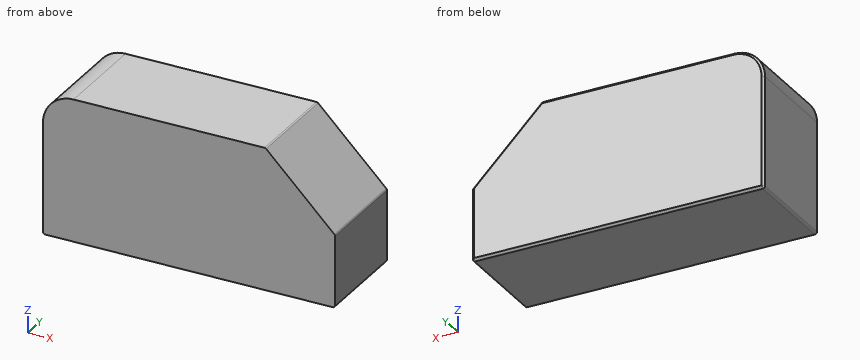
Autodesk Inventor part; units mm, degrees
ref_plane "YZ Plane" through (0, 0, 0) normal (1, 0, 0) x (0, 1, 0)
ref_plane "XZ Plane" through (0, 0, 0) normal (0, 1, 0) x (-1, 0, 0)
ref_plane "XY Plane" through (0, 0, 0) normal (0, 0, 1) x (1, 0, 0)
sketch "Sketch2" plane through (0, 0, 0) normal (0, 1, 0) x (-1, 0, 0)
  line L0 (-7.64, 0.08) -> (-7.64, -3.72)
  line L1 (-7.64, -3.72) -> (7.64, -3.72)
  line L2 (7.64, -3.72) -> (7.64, 2.12)
  arc A0 (7.64, 2.12) -> (6.04, 3.72) centre (6.04, 2.12) ccw
  line L3 (6.04, 3.72) -> (-4, 3.72)
  line L4 (-4, 3.72) -> (-7.64, 0.08)
  line L5 (0, -3.72) -> (0, 3.72) construction
  point P0 (0, 0)
  point P1 (0, 0)
  dimension "d0" = 7.44
  dimension "d1" = 15.28
  dimension "d2" = 1.6
  dimension "d3" = 3.64
  dimension "d4" = 3.64
extrude "Extrusion1" add sketch "Sketch2" along normal mid plane 5.2
fillet "Fillet1" radius 0.12 4 edges at (4, 0, 3.72) (7.64, 0, 0.08) (7.64, 0, -3.72) (-7.64, 0, -3.72)
chamfer "Chamfer2" distance 0.12 angle 45 10 edges at (-7.1714, 2.6, 3.2514) (-1.0449, 2.6, 3.72) (3.9962, 2.6, 3.7109) (5.82, 2.6, 1.9) (7.6309, 2.6, 0.0762) (7.64, 2.6, -1.7849) (7.6049, 2.6, -3.6849) (0, 2.6, -3.72) (-7.6049, 2.6, -3.6849) (-7.64, 2.6, -0.74)
equation "\"d4\" = d3"
properties part number "11030-LtBluishGray" material "ABS Plastic"
Can you work these out from the model? Positions are in its coordinate system, mm. Give positions to 0.01 mm unless a question says otherwise; leave off trailing zeros. Loops run counter-clockwise (first coordinate to the right, second up) from the corner with the lowest first, then second, coordinate; pieces in that order, holes last. Notation, with made-up numbers: (11.5, -33.75) - (36.5, -33.75) arc R22 cw to (36.5, -25.75) - close; hole circle Ø1 at (34, -31.5). An arc over 180 degrees is marked (long way). One line per item, written item: value.
(1) If we section it at B-B, the plane z = 1.5: List the corners of the cut face in (x, y) for me, plus the area to 3 significant figures.
Verdict:
outline: (-7.64, -2.6) - (6.22, -2.6) - (6.22, 2.48) - (6.05, 2.6) - (-7.52, 2.6) - (-7.64, 2.48) - close
area: 72.1 mm^2
(2) I need wall thicknesses on line 1 along X through (y, z) = (0.35, 1); line 2 along X through (y, z) = (-1.7, 0.25); line 3 along Z through (x, y) = (6, 0.15). Which ranges of each line are inside material? Lowest first, please.
Verdict:
line 1: -7.64 to 6.72
line 2: -7.64 to 7.47
line 3: -3.72 to 1.72
(3) I'm going to push a flat-ended pin straight in: pin 1 (3 mm diameter, centred on x = 4, y = -1.5, fed in from +Z). Where does the tip first touch, or does it pass through?
Verdict:
pin 1: z = 3.72
(4) If we section it at A-A, the plane y = 1.1: List the corners of the cut face in (x, z) for me, plus the area to 3 significant figures.
Verdict:
outline: (-7.64, -3.6) arc R0.12 ccw to (-7.52, -3.72) - (7.52, -3.72) arc R0.12 ccw to (7.64, -3.6) - (7.64, 0.03) arc R0.12 ccw to (7.6, 0.12) - (4.04, 3.68) arc R0.12 ccw to (3.95, 3.72) - (-6.04, 3.72) arc R1.6 ccw to (-7.64, 2.12) - close
area: 107 mm^2
